Part model, mm, in its own coordinate system. Round coordinates to 2 decimals unless told otherwise and drop trailing zeros. Loops run counter-clockwise (first coordinate to the right, second up) from the corner with the lowest first, then second, coordinate; pieces in that order, holes last. Notation, with made-up numbers: (-30, 86) -> (-24, 86) arc R8 cw to (-24, 98) -> close; hole circle Ø1 at (22.5, 70.25). An arc over 180 degrees is marked (long way). Answer as a JSON object with one key per item and string values. Group by question number.
from build123d import *

# Parameters (mm, degrees)
F0_W     = 15.875
F0_H     = 15.875
F0_W_2   = 14.2748
F0_H_2   = 14.2748
F1_DEPTH = 609.6
F3_DEPTH = 5.08
F4_R     = 1.7145
F5_DEPTH = 15.876


with BuildPart() as f1:
    # F0 (on Right) → F1 (new body, symmetric)
    with BuildSketch(Plane.YZ):
        Rectangle(F0_W, F0_H)
        Rectangle(F0_W_2, F0_H_2, mode=Mode.SUBTRACT)
    extrude(amount=F1_DEPTH, both=True)

    # F2 (on face) → F3 (cut)
    with BuildSketch(Plane(origin=(0, 0, -7.9375), x_dir=(1, 0, 0), z_dir=(0, 0, -1))):
        with BuildLine():
            Line((-17.145, 0), (17.145, 0))
            ThreePointArc((17.145, 0), (18.4920384182, 0.5579615818), (19.05, 1.905))
            ThreePointArc((19.05, 1.905), (18.4920384182, 3.2520384182), (17.145, 3.81))
            Line((17.145, 3.81), (-17.145, 3.81))
            ThreePointArc((-17.145, 3.81), (-18.4920384182, 3.2520384182), (-19.05, 1.905))
            ThreePointArc((-19.05, 1.905), (-18.4920384182, 0.5579615818), (-17.145, 0))
        make_face()
    extrude(amount=-F3_DEPTH, mode=Mode.SUBTRACT)

    # F4 (on face) → F5 (cut, through all)
    with BuildSketch(Plane(origin=(0, 0, -7.9375), x_dir=(1, 0, 0), z_dir=(0, 0, -1))):
        with Locations((-15.24, -3.175)):
            Circle(F4_R)
        with Locations((15.24, -3.175)):
            Circle(F4_R)
    extrude(amount=-F5_DEPTH, mode=Mode.SUBTRACT)


solid = f1.part
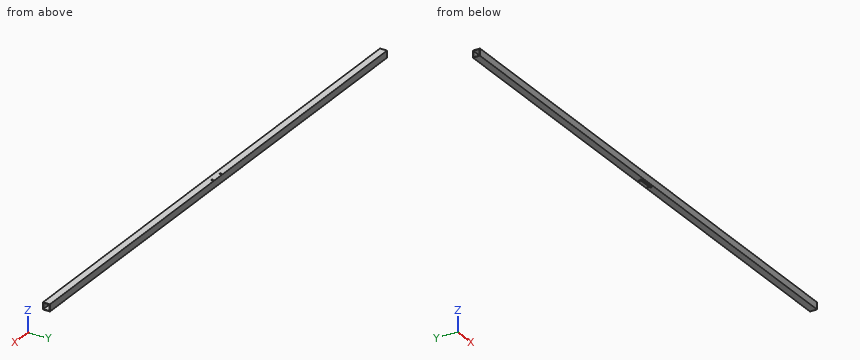
Item 1: Band-saw the part on A-A, the plane x = -315. List the corners of the cut face in (y, z), plus the area to 3 significant figures.
Item 2: Band-saw the part on B-B, the plane z = -3.5. List the corners of the cut face in (x, y), plus the area to 3 significant figures.
Item 3: Drill centre lines: line 1 (Y direction, x = 15.24, z = -7.6); line 2 (Y direction, x = -15.24, z = 7.5); line 3 (Z direction, x = 364.5, y = -1.5). Where is each one in solid material? Low to high.
Entries:
{
 "1": {"outline": "(-7.94, -7.94) -> (7.94, -7.94) -> (7.94, 7.94) -> (-7.94, 7.94) -> close; hole (-7.14, -7.14) -> (7.14, -7.14) -> (7.14, 7.14) -> (-7.14, 7.14) -> close", "area": "48.2 mm²"},
 "2": {"outline": "(-609.6, -7.94) -> (609.6, -7.94) -> (609.6, -7.14) -> (-609.6, -7.14) -> close; (-609.6, 7.14) -> (609.6, 7.14) -> (609.6, 7.94) -> (-609.6, 7.94) -> close", "area": "1,950 mm²"},
 "3": {"line 1": "-7.94 to -3.81, 0 to 1.46, 4.89 to 7.94", "line 2": "-7.94 to 1.46, 4.89 to 7.94", "line 3": "-7.94 to -7.14, 7.14 to 7.94"}
}
